For this review, use the dimensioned drawing (mm, ordinates from the lowest corner) and the shaded views. Coordinates: 2 decimals unless noted, no trailing zeros. Write each loop counter-clockwise with the first axis right and the second up, starting at its lowest first coordinate (ties: lowest second). Pieces come first, ordered by that corner, then holes.
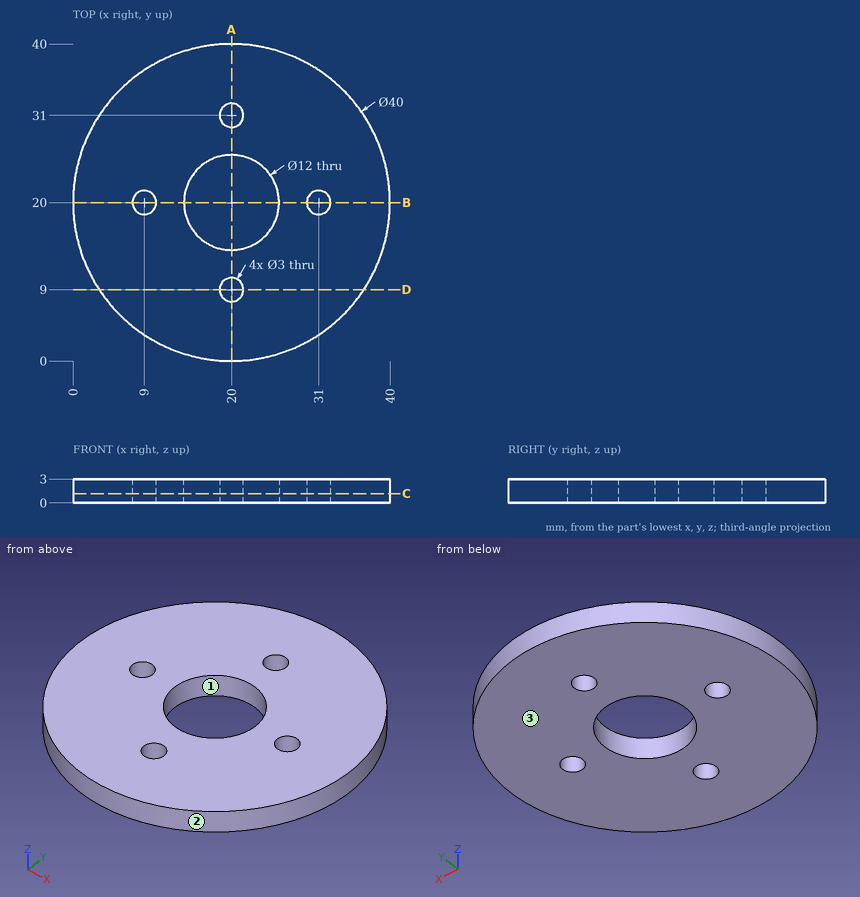
Item 1: Take a section at D-D, the plane y = 9. Write out the cut boundary in (x, z).
Solved:
outline: (3.3, 0) - (18.5, 0) - (18.5, 3) - (3.3, 3) - close; (21.5, 0) - (36.7, 0) - (36.7, 3) - (21.5, 3) - close
Item 2: To check wall thickness, follow line 1 along Y through (x, z) = (20, 1.1); line 2 along Y through (x, z) = (20.5, 2.7); line 3 along Y through (x, z) = (25.5, 0.75). State the ranges of each line that lie inside material, in increasing order.
Solved:
line 1: y = 0 to 7.5, 10.5 to 14, 26 to 29.5, 32.5 to 40
line 2: y = 0.01 to 7.59, 10.41 to 14.02, 25.98 to 29.59, 32.41 to 39.99
line 3: y = 0.77 to 17.6, 22.4 to 39.23
Item 3: Take a section at C-C, the plane z = 1.15. Write out the cut boundary in (x, y), plus the area to 3 significant figures.
Solved:
outline: circle Ø40 at (20, 20); hole circle Ø3 at (9, 20); hole circle Ø12 at (20, 20); hole circle Ø3 at (20, 9); hole circle Ø3 at (20, 31); hole circle Ø3 at (31, 20)
area: 1,120 mm2
Item 4: For pin 1 (3 mm diameter, centred on x = 15, y = 27, fed in from -Z); pin 2 (1 mm diameter, centred on x = 19, z = 2, fed in from -Y), all flat-tipped, find the tip position at first contact; note any pin that passes through.
Solved:
pin 1: stops at z = 0
pin 2: stops at y = 0.01
Item 5: Take a section at A-A, the plane x = 20. Write out the cut boundary in (y, z), plus the area to 3 significant figures.
Solved:
outline: (0, 0) - (7.5, 0) - (7.5, 3) - (0, 3) - close; (10.5, 0) - (14, 0) - (14, 3) - (10.5, 3) - close; (26, 0) - (29.5, 0) - (29.5, 3) - (26, 3) - close; (32.5, 0) - (40, 0) - (40, 3) - (32.5, 3) - close
area: 66.0 mm2
Item 6: Mouldability with a two-part tool opening along Y and no side actions: class the marked faces 1, 2 and 3 as pulls with the +Y half, pulls with the -Y half, needs draft (parallel to the pull), parting line crosses it, or undercut.
Solved:
face 1: undercut
face 2: parting line crosses it
face 3: needs draft
